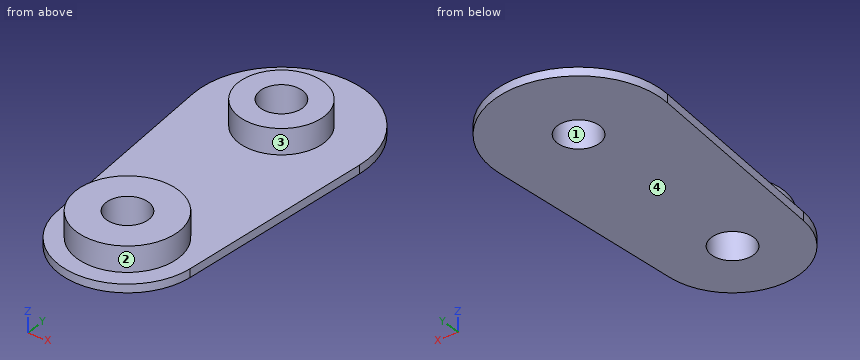
Autodesk Inventor part; units mm, degrees
ref_plane "YZ Plane" through (0, 0, 0) normal (1, 0, 0) x (0, 1, 0)
ref_plane "XZ Plane" through (0, 0, 0) normal (0, 1, 0) x (-1, 0, 0)
ref_plane "XY Plane" through (0, 0, 0) normal (0, 0, 1) x (1, 0, 0)
sketch "スケッチ1" plane through (0, 0, 0) normal (0, 0, 1) x (1, 0, 0)
  circle A0 centre (0, 0) radius 5
  circle A1 centre (0, -25) radius 10 construction
  spline S0 degree 4 number of poles 181
  arc A2 (-34.6019, -43.3635) -> (-36.604, -46.8264) centre (-35.6029, -45.0949) ccw
  line L0 (-36.604, -46.8264) -> (-35.6029, -45.0949) construction
  line L1 (-34.6019, -43.3635) -> (-35.6029, -45.0949) construction
  arc A3 (9.9747, -25.7104) -> (36.4435, -41.8861) centre (27.3937, -26.9509) ccw
  arc A4 (-34.6019, -43.3635) -> (-9.8865, -26.5022) centre (-26.2949, -28.9953) ccw
  line L2 (-4.899, 1) -> (-9.798, -23) construction
  line L3 (4.899, 1) -> (9.798, -23) construction
  circle A5 centre (0, 0) radius 2.5
  circle A6 centre (0, 0) radius 1.25
  circle A7 centre (0, -12) radius 1.25
  circle A8 centre (0, -12) radius 3
  circle A9 centre (0, -12) radius 4.255 construction
  line L4 (-3.817, -10.1196) -> (-8.9705, -20.5808) construction
  line L5 (3.817, -10.1196) -> (8.9705, -20.5808) construction
  circle A10 centre (0, -25) radius 7.025 construction
  circle A11 centre (0, -12) radius 4
  line L6 (17.164, -48.1611) -> (13.7217, -46.1237)
  line L7 (13.7217, -46.1237) -> (15.7591, -42.6814)
  line L8 (15.7591, -42.6814) -> (19.2014, -44.7188)
  line L9 (19.2014, -44.7188) -> (17.164, -48.1611)
  line L10 (-17.2597, -45.3722) -> (-13.9841, -43.0765)
  line L11 (-13.9841, -43.0765) -> (-11.6884, -46.3522)
  line L12 (-11.6884, -46.3522) -> (-14.964, -48.6478)
  line L13 (-14.964, -48.6478) -> (-17.2597, -45.3722)
  line L14 (15.4429, -47.1424) -> (17.4802, -43.7001) construction
  line L15 (-15.6219, -44.2243) -> (-13.3262, -47.5) construction
  arc A12 (38.5164, -45.3071) -> (36.4435, -41.8861) centre (37.48, -43.5966) ccw
  line L16 (38.5164, -45.3071) -> (37.48, -43.5966) construction
  line L17 (36.4435, -41.8861) -> (37.48, -43.5966) construction
  line L18 (-5.2079, 2.2776) -> (-3.9861, -12.3333)
  line L19 (4.9826, -0.4167) -> (3.9861, -12.3333)
  point P0 (38.0735, -45.574)
  point P1 (37.6323, -45.8368)
  point P2 (37.1929, -46.0956)
  point P3 (36.755, -46.3505)
  point P4 (36.3186, -46.6016)
  point P5 (35.8837, -46.8488)
  point P6 (35.4502, -47.0924)
  point P7 (35.0179, -47.3322)
  point P8 (34.5869, -47.5685)
  point P9 (34.157, -47.8012)
  point P10 (33.7283, -48.0304)
  point P11 (33.3005, -48.2561)
  point P12 (32.8738, -48.4785)
  point P13 (32.4479, -48.6974)
  point P14 (32.023, -48.9131)
  point P15 (31.5988, -49.1254)
  point P16 (31.1754, -49.3346)
  point P17 (30.7527, -49.5405)
  point P18 (30.3307, -49.7432)
  point P19 (29.9093, -49.9428)
  point P20 (29.4885, -50.1393)
  point P21 (29.0683, -50.3328)
  point P22 (28.6485, -50.5231)
  point P23 (28.2292, -50.7105)
  point P24 (27.8103, -50.8948)
  point P25 (27.3918, -51.0762)
  point P26 (26.9737, -51.2547)
  point P27 (26.5559, -51.4302)
  point P28 (26.1384, -51.6028)
  point P29 (25.7211, -51.7725)
  point P30 (25.3041, -51.9393)
  point P31 (24.8874, -52.1033)
  point P32 (24.4708, -52.2644)
  point P33 (24.0544, -52.4227)
  point P34 (23.6381, -52.5782)
  point P35 (23.2219, -52.731)
  point P36 (22.8059, -52.8809)
  point P37 (22.39, -53.028)
  point P38 (21.9741, -53.1724)
  point P39 (21.5582, -53.3141)
  point P40 (21.1424, -53.453)
  point P41 (20.7266, -53.5892)
  point P42 (20.3109, -53.7226)
  point P43 (19.8951, -53.8534)
  point P44 (19.4793, -53.9814)
  point P45 (19.0635, -54.1068)
  point P46 (18.6476, -54.2294)
  point P47 (18.2317, -54.3494)
  point P48 (17.8157, -54.4666)
  point P49 (17.3997, -54.5812)
  point P50 (16.9836, -54.6931)
  point P51 (16.5674, -54.8024)
  point P52 (16.1511, -54.909)
  point P53 (15.7347, -55.0129)
  point P54 (15.3182, -55.1141)
  point P55 (14.9017, -55.2128)
  point P56 (14.485, -55.3087)
  point P57 (14.0682, -55.402)
  point P58 (13.6513, -55.4927)
  point P59 (13.2343, -55.5807)
  point P60 (12.8172, -55.666)
  point P61 (12.3999, -55.7487)
  point P62 (11.9826, -55.8288)
  point P63 (11.5651, -55.9062)
  point P64 (11.1476, -55.981)
  point P65 (10.7299, -56.0532)
  point P66 (10.3121, -56.1227)
  point P67 (9.8942, -56.1895)
  point P68 (9.4762, -56.2538)
  point P69 (9.0581, -56.3154)
  point P70 (8.6399, -56.3743)
  point P71 (8.2216, -56.4306)
  point P72 (7.8032, -56.4843)
  point P73 (7.3847, -56.5353)
  point P74 (6.9661, -56.5837)
  point P75 (6.5474, -56.6295)
  point P76 (6.1287, -56.6726)
  point P77 (5.7099, -56.7131)
  point P78 (5.2911, -56.751)
  point P79 (4.8721, -56.7862)
  point P80 (4.4532, -56.8187)
  point P81 (4.0341, -56.8487)
  point P82 (3.6151, -56.876)
  point P83 (3.196, -56.9006)
  point P84 (2.7768, -56.9226)
  point P85 (2.3577, -56.942)
  point P86 (1.9385, -56.9588)
  point P87 (1.5194, -56.9728)
  point P88 (1.1002, -56.9843)
  point P89 (0.681, -56.9931)
  point P90 (0.2619, -56.9993)
  point P91 (-0.1572, -57.0028)
  point P92 (-0.5763, -57.0037)
  point P93 (-0.9954, -57.002)
  point P94 (-1.4144, -56.9976)
  point P95 (-1.8334, -56.9906)
  point P96 (-2.2523, -56.9809)
  point P97 (-2.6711, -56.9686)
  point P98 (-3.0898, -56.9537)
  point P99 (-3.5085, -56.9361)
  point P100 (-3.9271, -56.9159)
  point P101 (-4.3456, -56.893)
  point P102 (-4.764, -56.8675)
  point P103 (-5.1822, -56.8394)
  point P104 (-5.6004, -56.8086)
  point P105 (-6.0184, -56.7752)
  point P106 (-6.4363, -56.7391)
  point P107 (-6.854, -56.7004)
  point P108 (-7.2716, -56.6591)
  point P109 (-7.689, -56.6152)
  point P110 (-8.1063, -56.5686)
  point P111 (-8.5234, -56.5194)
  point P112 (-8.9403, -56.4675)
  point P113 (-9.357, -56.413)
  point P114 (-9.7736, -56.3559)
  point P115 (-10.1899, -56.2961)
  point P116 (-10.6061, -56.2337)
  point P117 (-11.022, -56.1687)
  point P118 (-11.4378, -56.1011)
  point P119 (-11.8533, -56.0308)
  point P120 (-12.2686, -55.9579)
  point P121 (-12.6837, -55.8823)
  point P122 (-13.0985, -55.8041)
  point P123 (-13.5132, -55.7233)
  point P124 (-13.9276, -55.6399)
  point P125 (-14.3417, -55.5538)
  point P126 (-14.7557, -55.4651)
  point P127 (-15.1694, -55.3738)
  point P128 (-15.5828, -55.2798)
  point P129 (-15.996, -55.1832)
  point P130 (-16.409, -55.084)
  point P131 (-16.8217, -54.9821)
  point P132 (-17.2342, -54.8776)
  point P133 (-17.6465, -54.7704)
  point P134 (-18.0585, -54.6606)
  point P135 (-18.4703, -54.5482)
  point P136 (-18.8818, -54.4331)
  point P137 (-19.2932, -54.3154)
  point P138 (-19.7043, -54.195)
  point P139 (-20.1152, -54.0719)
  point P140 (-20.5259, -53.9462)
  point P141 (-20.9364, -53.8179)
  point P142 (-21.3468, -53.6868)
  point P143 (-21.7569, -53.5531)
  point P144 (-22.1669, -53.4167)
  point P145 (-22.5767, -53.2776)
  point P146 (-22.9864, -53.1358)
  point P147 (-23.3959, -52.9913)
  point P148 (-23.8053, -52.8441)
  point P149 (-24.2147, -52.6941)
  point P150 (-24.6239, -52.5414)
  point P151 (-25.0331, -52.386)
  point P152 (-25.4422, -52.2278)
  point P153 (-25.8514, -52.0669)
  point P154 (-26.2605, -51.9031)
  point P155 (-26.6697, -51.7366)
  point P156 (-27.0789, -51.5672)
  point P157 (-27.4882, -51.395)
  point P158 (-27.8976, -51.2199)
  point P159 (-28.3071, -51.0419)
  point P160 (-28.7169, -50.8611)
  point P161 (-29.1269, -50.6773)
  point P162 (-29.5371, -50.4905)
  point P163 (-29.9476, -50.3008)
  point P164 (-30.3585, -50.1081)
  point P165 (-30.7698, -49.9123)
  point P166 (-31.1815, -49.7134)
  point P167 (-31.5937, -49.5114)
  point P168 (-32.0065, -49.3063)
  point P169 (-32.4199, -49.0979)
  point P170 (-32.8339, -48.8863)
  point P171 (-33.2488, -48.6714)
  point P172 (-33.6644, -48.4532)
  point P173 (-34.081, -48.2315)
  point P174 (-34.4985, -48.0064)
  point P175 (-34.9171, -47.7778)
  point P176 (-35.3368, -47.5455)
  point P177 (-35.7578, -47.3096)
  point P178 (-36.1802, -47.0699)
  point P179 (-4.9826, -0.4167)
  dimension "d0" = 10
  dimension "d1" = 20
  dimension "d2" = 2
  dimension "d3" = 180
  dimension "d4" = 25
  dimension "d5" = 5
  dimension "d6" = 2.5
  dimension "d7" = 2.5
  dimension "d8" = 6
  dimension "d9" = 8.51
  dimension "d10" = 12
  dimension "d11" = 14.05
  dimension "d12" = 8
  dimension "d13" = 4
  dimension "d14" = 4
  dimension "d15" = 4
  dimension "d16" = 4
  dimension "d17" = 16.5967
  dimension "d18" = 17.4631
  dimension "d19" = 18.5967
  dimension "d20" = 19.4631
  dimension "d21" = 20
  dimension "d22" = 2
  dimension "d23" = 180
  dimension "d24" = 20
extrude "押し出し1" add sketch "スケッチ1" along normal blind 0.5 contours A0 | L19 A11 L18 A0 | A11
extrude "押し出し2" add sketch "スケッチ1" along normal blind 2 contours A5 | A8
equation "\"d6\" = d7"
properties part number "揺動節抑え" material "アルミニウム 2014-T4"
The listing builds one solid part. Answer for the finished solid, in the listing's coordinates (mm). Face numbers are marked on the shaded views. A direction names the side the tool comes from. Coordinates: 2 decimals unless noted, no trailing zeros. Write each loop counter-clockwise with the first axis right and the second up, starting at its lowest first coordinate (ties: lowest second). Pieces come first, ordered by that corner, then holes. Notation, with made-up numbers: (3, 11.5) - (38, 11.5) arc R31 ccw to (38, 39.5) - close; hole circle Ø1 at (-39, 9.5). An arc over 180 degrees is marked (long way). Return JSON: item names as keys, results as strings. Group by question number.
Q1. For a pull along Y with two mould halves and no side action, classify the marked faces 3 and 4 as +Y half, -Y half, draft (parallel to the pull), parting line (faces both ways), or undercut.
Q2. Find the intervals of material crossed by line 1 along Y through (x, z) = (0, 1.15); line 2 along Y through (x, z) = (0.75, 0.35); line 3 along Y through (x, z) = (0.75, 0.8), in increasing order. Write a range as [from, to].
Q3. The part is cut by section B-B on x = 0. Write down the section's boundary in (y, z).
Q4. The part is cut by section C-C on z = 0.75. Write down the section's boundary in (x, y), and give its area (3 significant figures).
Q5. A flat-ended cylindrical pin translates along its axis: pin 1 Ø2 at (x, y) = (0, 0) entering from -Z. Find the tip coordinate at first contact, or state that the pin passes through.
Q6. The part is cut by section D-D on x = -1.75. Write down the section's boundary in (y, z), and give its area (3 significant figures).
Q7. Which of the six approach directions +Z, -Z, +X, -X, +Y, -Y give full straight-line access (tool end or side, diameter ignored) to the marked faces 1 and 2?
Q8. The part is cut by section A-A on y = 0. Write down the section's boundary in (x, z).
Evaluation:
{
 "1": {"face 3": "undercut", "face 4": "draft"},
 "2": {"line 1": "y = [-15, -13.25], [-10.75, -9], [-2.5, -1.25], [1.25, 2.5]", "line 2": "y = [-15.93, -13], [-11, -1], [1, 4.94]", "line 3": "y = [-14.9, -13], [-11, -9.1], [-2.38, -1], [1, 2.38]"},
 "3": {"outline": "(-16, 0) - (-13.25, 0) - (-13.25, 2) - (-15, 2) - (-15, 0.5) - (-16, 0.5) - close; (-10.75, 0) - (-1.25, 0) - (-1.25, 2) - (-2.5, 2) - (-2.5, 0.5) - (-9, 0.5) - (-9, 2) - (-10.75, 2) - close; (1.25, 0) - (5, 0) - (5, 0.5) - (2.5, 0.5) - (2.5, 2) - (1.25, 2) - close"},
 "4": {"outline": "circle Ø6 at (0, -12); circle Ø5 at (0, 0); hole circle Ø2.5 at (0, -12); hole circle Ø2.5 at (0, 0)", "area": "38.1 mm2"},
 "5": {"pin 1": "passes through"},
 "6": {"outline": "(-15.6, 0) - (4.68, 0) - (4.68, 0.5) - (1.79, 0.5) - (1.79, 2) - (-1.79, 2) - (-1.79, 0.5) - (-9.56, 0.5) - (-9.56, 2) - (-14.44, 2) - (-14.44, 0.5) - (-15.6, 0.5) - close", "area": "22.8 mm2"},
 "7": {"face 1": "+Z, -Z", "face 2": "+Z"},
 "8": {"outline": "(-5, 0) - (-1.25, 0) - (-1.25, 2) - (-2.5, 2) - (-2.5, 0.5) - (-5, 0.5) - close; (1.25, 0) - (5, 0) - (5, 0.5) - (2.5, 0.5) - (2.5, 2) - (1.25, 2) - close"}
}
